Model file for the job. Use its own axes, mm. A direction names the side the tool comes from. Coordinates: 2 decimals unless noted, no trailing zeros. Loops run counter-clockwise (first coordinate to the right, second up) from the corner with the lowest first, then second, coordinate; pieces in that order, holes last. Notation, with made-up numbers: M 83,-22.5 L 121,-22.5 A16 ccw 121,-15.5 Z; hole C 4.5,26 d5. An arc over 180 degrees is marked long. One line per question, with ' | ' between items. Start each with the question number.
```python
from build123d import *

# Parameters (mm, degrees)
SKETCH2_W           = 80
SKETCH2_H           = 80
BOSS_EXTRUDE1_DEPTH = 4
SKETCH3_R           = 10
CUT_EXTRUDE1_DEPTH  = 4
SKETCH4_R           = 1.75
CUT_EXTRUDE2_DEPTH  = 10
SKETCH7_W           = 80
SKETCH7_H           = 39.2
BOSS_EXTRUDE3_DEPTH = 4
SKETCH8_W           = 20
SKETCH8_H           = 80
BOSS_EXTRUDE4_DEPTH = 4
SKETCH9_R           = 2.5
CUT_EXTRUDE3_DEPTH  = 4
FILLET1_R           = 5


with BuildPart() as part:
    # Sketch2 → Boss-Extrude1 (new body)
    with BuildSketch(Plane(origin=(0, 0, 0), x_dir=(1, 0, 0), z_dir=(0, 1, 0))):
        Rectangle(SKETCH2_W, SKETCH2_H)
    extrude(amount=BOSS_EXTRUDE1_DEPTH)

    # Sketch3 → Cut-Extrude1 (cut)
    with BuildSketch(Plane(origin=(0, 4, 0), x_dir=(1, 0, 0), z_dir=(0, 1, 0))):
        with Locations(Location((0, -7.5, 0), (0, 0, 270))):
            Circle(SKETCH3_R)
    extrude(amount=-CUT_EXTRUDE1_DEPTH, mode=Mode.SUBTRACT)

    # Sketch4 → Cut-Extrude2 (cut)
    with BuildSketch(Plane(origin=(0, 4, 0), x_dir=(1, 0, 0), z_dir=(0, 1, 0))):
        with Locations(Location((-28.231866882, -35.612184397, 0), (0, 0, 270))):
            Circle(SKETCH4_R)
        with Locations(Location((27.768133118, -35.612184397, 0), (0, 0, 270))):
            Circle(SKETCH4_R)
        with Locations(Location((19.768133118, 34.387815603, 0), (0, 0, 270))):
            Circle(SKETCH4_R)
        with Locations(Location((-20.231866882, 34.387815603, 0), (0, 0, 270))):
            Circle(SKETCH4_R)
    extrude(amount=-CUT_EXTRUDE2_DEPTH, mode=Mode.SUBTRACT)

    # Sketch7 → Boss-Extrude3 (add)
    with BuildSketch(Plane.ZY.offset(40)):
        with Locations((0, 19.6)):
            Rectangle(SKETCH7_W, SKETCH7_H)
    boss_extrude3 = extrude(amount=BOSS_EXTRUDE3_DEPTH)

    # Mirror2: Boss-Extrude3 across plane
    add(boss_extrude3.mirror(Plane(origin=(0, 0, 0), x_dir=(0, 0, 1), z_dir=(1, 0, 0))))

    # Sketch8 → Boss-Extrude4 (add)
    with BuildSketch(Plane(origin=(0, 39.2, 0), x_dir=(1, 0, 0), z_dir=(0, 1, 0))):
        with Locations((-50, 0)):
            Rectangle(SKETCH8_W, SKETCH8_H)
    boss_extrude4 = extrude(amount=-BOSS_EXTRUDE4_DEPTH)

    # Mirror3: Boss-Extrude4 across plane
    add(boss_extrude4.mirror(Plane(origin=(0, 0, 0), x_dir=(0, 0, 1), z_dir=(1, 0, 0))))

    # Sketch9 → Cut-Extrude3 (cut)
    with BuildSketch(Plane(origin=(0, 39.2, 0), x_dir=(1, 0, 0), z_dir=(0, 1, 0))):
        with Locations(Location((-52, -25, 0), (0, 0, 270))):
            Circle(SKETCH9_R)
        with Locations(Location((-52, 25, 0), (0, 0, 90))):
            Circle(SKETCH9_R)
        with Locations(Location((52, 25, 0), (0, 0, 270))):
            Circle(SKETCH9_R)
        with Locations(Location((52, -25, 0), (0, 0, 90))):
            Circle(SKETCH9_R)
    extrude(amount=-CUT_EXTRUDE3_DEPTH, mode=Mode.SUBTRACT)

    # Fillet1
    fillet1_edges = [part.edges().sort_by_distance(p)[0] for p in [
        (40, 4, 0),
        (-40, 4, 0),
        (-40, 39.2, 0),
        (-44, 0, 0),
        (40, 39.2, 0),
        (44, 0, 0),
        (-44, 35.2, 0),
        (-60, 37.2, -40),
        (-60, 37.2, 40),
        (44, 35.2, 0),
        (60, 37.2, 40),
        (60, 37.2, -40),
    ]]
    fillet(fillet1_edges, radius=FILLET1_R)


solid = part.part
```
(1) Pin check, flat tips, straight feed: P1, Ø4, axis at x = 27.77, z = 35.61, coming from the -Y side; P2, Ø3, axis at x = 19.77, z = -34.39, coming from the +Y side; P3, Ø1, axis at x = 37, z = -7, coming from the +Y side; P4, Ø5.5, axis at x = -20.23, z = -34.39, coming from the +Y side. Stop position of each tip, or through.
(2) Band-saw the part on B-B on z = 25. Write the cut outline in (x, y).
(3) Drill centre lines: line 1 (X direction, y = 16, z = 0); line 2 (X direction, y = 37.3, z = 25); line 3 (X direction, y = 2.5, z = 36.5). Where is each one in solid material? Low to high. Write a range as [from, to].
(4) 3-axis set-ups, long thin cutter, end or side, ignore diameter. For faces 4 (the face through (7, 4, -1)), 5 (the face through (-58, 37, 39)), 6 (the face through (-44, 18, -1)): which of +Z, -Z, +X, -X, +Y, -Y reach the whole face in a straight line?
(5) Band-saw the part on C-C on z = 15.5. Write the cut outline in (x, y).
(6) Band-saw the part on A-A on x = -52. Write the cut outline in (y, z).
(7) Two-plate mould, pull along Z, no slides. Class faces 1 (the face through (41.5, 37.77, 0.56)), 2 (the face through (-54.44, 37.23, 24.46)), 3 (the face through (0, 2, 40)): pulls with the +Z half, pulls with the -Z half, needs draft (parallel to the pull), parting line crosses it, or undercut.
(8) Band-saw the part on D-D on x = 0. Write the cut outline in (y, z), then the cut area to 3 significant figures.
Computed values:
1) P1: y = 0 | P2: through | P3: y = 4.67 | P4: y = 4
2) outline: M -60,35.2 L -54.5,35.2 L -54.5,39.2 L -60,39.2 Z; M -49.5,35.2 L -49,35.2 A5 cw -44,30.2 L -44,5 A5 ccw -39,0 L 39,0 A5 ccw 44,5 L 44,30.2 A5 cw 49,35.2 L 49.5,35.2 L 49.5,39.2 L 45,39.2 A5 ccw 40,34.2 L 40,9 A5 cw 35,4 L -35,4 A5 cw -40,9 L -40,34.2 A5 ccw -45,39.2 L -49.5,39.2 Z; M 54.5,35.2 L 60,35.2 L 60,39.2 L 54.5,39.2 Z
3) line 1: [-44, -40], [40, 44] | line 2: [-60, -54.5], [-49.5, -41.08], [41.08, 49.5], [54.5, 60] | line 3: [-43.33, -29.74], [-26.72, 26.26], [29.28, 43.33]
4) face 4: +Z, -Z, +Y | face 5: +Z, -X, +Y, -Y | face 6: +Z, -Z, -X, -Y
5) outline: M -60,35.2 L -49,35.2 A5 cw -44,30.2 L -44,5 A5 ccw -39,0 L -6,0 L -6,4 L -35,4 A5 cw -40,9 L -40,34.2 A5 ccw -45,39.2 L -60,39.2 Z; M 6,0 L 39,0 A5 ccw 44,5 L 44,30.2 A5 cw 49,35.2 L 60,35.2 L 60,39.2 L 45,39.2 A5 ccw 40,34.2 L 40,9 A5 cw 35,4 L 6,4 Z
6) outline: M 35.2,-40 L 39.2,-40 L 39.2,-27.5 L 35.2,-27.5 Z; M 35.2,-22.5 L 39.2,-22.5 L 39.2,22.5 L 35.2,22.5 Z; M 35.2,27.5 L 39.2,27.5 L 39.2,40 L 35.2,40 Z
7) face 1: needs draft | face 2: undercut | face 3: pulls with the +Z half
8) outline: M 0,-40 L 4,-40 L 4,-2.5 L 0,-2.5 Z; M 0,17.5 L 4,17.5 L 4,40 L 0,40 Z | area: 240 mm^2
